Design review of the part built by this model. Coordinates are the model's own, in mm. A direction names the side the tool comes from. Coordinates: 2 decimals unless noted, no trailing zeros. Loops run counter-clockwise (first coordinate to the right, second up) from the corner with the lowest first, then second, coordinate; pieces in that order, holes last. Notation, with made-up numbers: M 87,70.5 L 137,70.5 A16 ccw 137,101.5 Z; hole C -9.5,63.5 d3. An arc over 180 degrees is marked long. Put each result on its own line as item: value. Start each with the question number.
(1) Take a section at A-A, the plane x = 0. Give the boundary of the cut face in (y, z), then the cut area to 3 significant figures.
(2) For faces 5 (the flat face through (-50, -1, 21)), 6 (the flat face through (90, -1, 5)), 7 (the flat face through (50, -1, 21)), list the 3-axis set-ups (+Z, -Z, +X, -X, +Y, -Y) from which the entire face can be reached by the end or side of a thin tool; tool diameter is ignored.
(3) Take a section at C-C, the plane y = 15. Count the separate pieces of the cut face and the enclosed holes in it, then the cut area to 3 significant figures.
(4) The part is to be moulded in two halves that separate along X. For faces 1 (the cylindrical face through (-62.31, 15.96, 6.06)), 2 (the cylindrical face through (-23.977, 1.055, 16.224)), 3 (the flat face through (-73, 1, 10)), 4 (the flat face through (-90, -1, 5)), say which applies: +X half, -X half, draft (parallel to the pull), parting line (faces both ways), or undercut.
(5) Clearance check with flat-ended pins moving along their axes: pin 1 (8 mm diameter, centred on x = 60, y = -15, fed in from -Z); pin 2 (4 mm diameter, centred on x = 48, y = 1, fed in from -Z); pin 3 (4.5 mm diameter, centred on x = 60, y = 15, fed in from -Z) (3 decimals); pin 4 (4 mm diameter, centred on y = -13.5, z = 7.5, fed in from -X). State where each tip first meets the part, or that it passes through.
(6) For probe 1 along Y at (x, z) = (60, 5); probe 2 along X at (y, z) = (15, 5) (3 decimals); probe 3 along X at (y, z) = (15, 7.25) (3 decimals), list the stretches that pass through material, from the lowest coordinate up. Write a range as [from, to].
```python
from build123d import *

# Parameters (mm, degrees)
F0_W           = 190
F0_H           = 75
F1_DEPTH       = 10
F2_W           = 100
F2_H           = 75
F3_DEPTH       = 22
F4_R           = 24
F5_DEPTH       = 32.001
F6_SIZE        = 9.99999
F8_D           = 5
F8_CSINK_D     = 9
F8_CSINK_ANGLE = 90


# Not quite as in the source:
# - a fillet or chamfer is up to 0.001 mm smaller than in the source, because OpenCascade refuses the exact size


with BuildPart() as f1:
    # F0 (on Top) → F1 (new body)
    with BuildSketch(Plane.XY):
        Rectangle(F0_W, F0_H)
    extrude(amount=F1_DEPTH)

    # F2 (on face) → F3 (join)
    with BuildSketch(Plane.XY.offset(10)):
        Rectangle(F2_W, F2_H)
    extrude(amount=F3_DEPTH)

    # F4 (on face) → F5 (cut, through all)
    with BuildSketch(Plane.XY.offset(32)):
        Circle(F4_R)
    extrude(amount=-F5_DEPTH, mode=Mode.SUBTRACT)

    # F6 (size 10 in the source; OpenCascade refuses exactly that, so slightly less here)
    f6_edges = [f1.edges().sort_by_distance(p)[0] for p in [
        (95, 0, 0),
        (-95, 0, 0),
        (0, 37.5, 0),
        (0, -37.5, 0),
    ]]
    chamfer(f6_edges, length=F6_SIZE)

    # F8 (through all)
    with Locations(Plane(origin=(0, 0, 0), x_dir=(1, 0, 0), z_dir=(0, 0, -1))):
        with Locations((-60, 15), (-60, -15), (60, 15), (60, -15)):
            CounterSinkHole(F8_D / 2, F8_CSINK_D / 2, counter_sink_angle=F8_CSINK_ANGLE)


solid = f1.part
```
Computed values:
1. outline: M -37.5,10 L -27.5,0 L -24,0 L -24,32 L -37.5,32 Z; M 24,0 L 27.5,0 L 37.5,10 L 37.5,32 L 24,32 Z
1. area: 764 mm^2
2. face 5: +Z, -X, +Y, -Y
2. face 6: -Z, +X, +Y, -Y
2. face 7: +Z, +X, +Y, -Y
3. separate pieces: 4
3. enclosed holes: 0
3. area: 2,690 mm^2
4. face 1: undercut
4. face 2: undercut
4. face 3: draft
4. face 4: -X half
5. pin 1: stops at z = 0.5
5. pin 2: stops at z = 0
5. pin 3: passes through
5. pin 4: stops at x = -94.5
6. probe 1: y = [-32.5, -17.5], [-12.5, 12.5], [17.5, 32.5]
6. probe 2: x = [-90, -62.5], [-57.5, -18.735], [18.735, 57.5], [62.5, 90]
6. probe 3: x = [-92.25, -62.5], [-57.5, -18.735], [18.735, 57.5], [62.5, 92.25]
